The listing builds one solid part. Answer for the finished solid, in the listing's coordinates (mm). A direction names the side the tool comes from. Give positions to 0.01 mm unless a question says otherwise; leave off trailing zeros. Write each loop counter-clockwise with the first axis right and the second up, starting at its lowest first coordinate (ties: lowest second). Pieces come first, ordered by that corner, then holes.
```python
from build123d import *

# Parameters (mm, degrees)
BOSS_EXTRUDE1_DEPTH = 101.6
SKETCH2_R           = 3.175
CUT_EXTRUDE1_DEPTH  = 101.6
SKETCH3_R           = 3.175
SKETCH3_R_2         = 2.38125
CUT_EXTRUDE2_DEPTH  = 101.6
SKETCH4_W           = 29.676804306
SKETCH4_H           = 30.942193328
CUT_EXTRUDE3_DEPTH  = 101.6


with BuildPart() as part:
    # Sketch1 → Boss-Extrude1 (new body)
    with BuildSketch(Plane(origin=(0, 0, 0), x_dir=(0, 0, -1), z_dir=(1, 0, 0))):
        Polygon((0, 0), (0, 25.4), (-1.5875, 25.4), (-1.5875, 1.5875), (-25.4, 1.5875), (-25.4, 0), align=None)
    boss_extrude1 = extrude(amount=BOSS_EXTRUDE1_DEPTH)

    # Sketch2 → Cut-Extrude1 (cut)
    with BuildSketch(Plane(origin=(0, 1.5875, 0), x_dir=(1, 0, 0), z_dir=(0, 1, 0))):
        with Locations((12.7, -13.49375)):
            Circle(SKETCH2_R)
        with Locations((88.9, -13.49375)):
            Circle(SKETCH2_R)
    cut_extrude1 = extrude(amount=-CUT_EXTRUDE1_DEPTH, mode=Mode.SUBTRACT)

    # Sketch3 → Cut-Extrude2 (cut)
    with BuildSketch(Plane.XY.offset(1.5875)):
        with Locations((69.85, 12.7)):
            Circle(SKETCH3_R)
        with Locations((6.35, 17.4625)):
            Circle(SKETCH3_R_2)
        with Locations((6.35, 7.9375)):
            Circle(SKETCH3_R_2)
    cut_extrude2 = extrude(amount=-CUT_EXTRUDE2_DEPTH, mode=Mode.SUBTRACT)

    # Mirror1: Boss-Extrude1, Cut-Extrude1, Cut-Extrude2 across plane
    add(boss_extrude1.mirror(Plane(origin=(101.6, 0, 0), x_dir=(1, 0, 0), z_dir=(0, 0, 1))))
    add(cut_extrude1.mirror(Plane(origin=(101.6, 0, 0), x_dir=(1, 0, 0), z_dir=(0, 0, 1))), mode=Mode.SUBTRACT)
    add(cut_extrude2.mirror(Plane(origin=(101.6, 0, 0), x_dir=(1, 0, 0), z_dir=(0, 0, 1))), mode=Mode.SUBTRACT)

    # Sketch4 → Cut-Extrude3 (cut)
    with BuildSketch(Plane.ZY):
        with Locations((14.838402153, 15.471096664)):
            Rectangle(SKETCH4_W, SKETCH4_H)
    extrude(amount=-CUT_EXTRUDE3_DEPTH, mode=Mode.SUBTRACT)


solid = part.part
```
Item 1: A cutting plane is placed at A-A, the plane x = 88.9. Give the vertices of the cut face in (y, z), plus the area to 3 significant figures.
Conclusion:
outline: (0, -25.4) - (1.59, -25.4) - (1.59, -16.67) - (0, -16.67) - close; (0, -10.32) - (1.59, -10.32) - (1.59, -1.59) - (25.4, -1.59) - (25.4, 0) - (0, 0) - close
area: 68.0 mm2
Item 2: Consider probe 1 along Y at (x, z) = (6.35, -0.5); probe 2 along Y at (x, z) = (69.85, -0.9) (3 decimals); probe 3 along Z at (x, y) = (88.9, 1.25). Determine where each line is inside the solid, lowest interval first.
Conclusion:
probe 1: y = 0 to 5.56, 10.32 to 15.08, 19.84 to 25.4
probe 2: y = 0 to 9.525, 15.875 to 25.4
probe 3: z = -25.4 to -16.67, -10.32 to 0
Item 3: A cutting plane is placed at C-C, the plane x = 6.35. Give the vertices of the cut face in (y, z), plus the area to 3 significant figures.
Conclusion:
outline: (0, -25.4) - (1.59, -25.4) - (1.59, -1.59) - (5.56, -1.59) - (5.56, 0) - (0, 0) - close; (10.32, -1.59) - (15.08, -1.59) - (15.08, 0) - (10.32, 0) - close; (19.84, -1.59) - (25.4, -1.59) - (25.4, 0) - (19.84, 0) - close
area: 63.0 mm2
Item 4: A cutting plane is placed at B-B, the plane y = 12.7. Give the vertices of the cut face in (x, z) (1 decimal), plus the area to 3 significant figures.
Conclusion:
outline: (0, -1.6) - (66.7, -1.6) - (66.7, 0) - (0, 0) - close; (73, -1.6) - (101.6, -1.6) - (101.6, 0) - (73, 0) - close
area: 151 mm2
Item 5: A cutting plane is placed at D-D, the plane z = -11.75. Give the vertices of the cut face in (x, y).
Conclusion:
outline: (0, 0) - (10.05, 0) - (10.05, 1.59) - (0, 1.59) - close; (15.35, 0) - (86.25, 0) - (86.25, 1.59) - (15.35, 1.59) - close; (91.55, 0) - (101.6, 0) - (101.6, 1.59) - (91.55, 1.59) - close
Item 6: Each of these flat-tipped pins is pushed along its axis until it touches: P1, Ø3, axis at x = 33, z = -11, coming from the +Y side; P2, Ø5.5, axis at x = 6.35, y = 7.94, coming from the -Z side; P3, Ø4, axis at x = 69.85, y = 12.7, coming from the -Z side (3 decimals). Where does it stop, or does it pass through?
Conclusion:
P1: stops at y = 1.59
P2: stops at z = -1.59
P3: passes through
Item 7: Determine the mould class of faces 3 (the face through (50, 0, -13)), 4 (the face through (0, 7, -1)), 5 (the face through (4.595, 19.072, -0.805)), 6 (the face through (67.33, 10.77, -0.8)) for opening direction Y: pulls with the +Y half, pulls with the -Y half, needs draft (parallel to the pull), parting line crosses it, or undercut.
Conclusion:
face 3: pulls with the -Y half
face 4: needs draft
face 5: undercut
face 6: undercut
Item 8: Which of the six approach directions +Z, -Z, +X, -X, +Y, -Y give full straight-line access (tool end or side, diameter ignored) to faces 1 (the face through (50, 14, -1.588)), 2 (the face through (12.012, 0.805, -16.593))?
Conclusion:
face 1: -Z, +X, -X, +Y
face 2: +Y, -Y
